Drawing for the job (mm, zero at the part's lowest x, y, z). A direction names the side the tool comes from. Give positions to 0.01 mm unless a question says otherwise; leave off trailing zeros. Order: outer loops, then holes, each group sorted by start corner. A loop starts at its lowest first (then second) coordinate and runs counter-clockwise, first axis right, second up. Notation, with made-up numbers: (-24.5, -40) -> (-3.5, -40) arc R25 cw to (-3.5, -20) -> close; hole circle Ø5 at (4, 65). An arc over 180 degrees is marked (long way). One line per item, written item: value. Start each with the question number.
(1) Pin check, flat tips, straight feed: pin 1 (17.5 mm diameter, centred on x = 24, z = 24.5, fed in from +Y); pin 2 (6.5 mm diameter, centred on x = 40.5, y = 7.5, fed in from +Z); pin 3 (4.5 mm diameter, centred on x = 7.5, y = 7.5, fed in from -Z); pin 4 (7.5 mm diameter, centred on y = 5, z = 12, fed in from -X). Stop position of each tip, or through.
(2) Saw through at D-D on x = 7.5. Give the cut face in (y, z), plus the area to 3 significant figures.
(3) Probe line 1 (Y direction, x = 40.5, z = 3.35); line 2 (Z direction, x = 24, y = 9); line 3 (Y direction, x = 40, z = 3). List the from-to ranges inside material, lowest first.
(4) Saw through at A-A on y = 43.5. Give the cut face in (x, z), plus the area to 3 significant figures.
(5) Which spindle directions (+Z, -Z, +X, -X, +Y, -Y) get a long thin tool onto all of the face, cutting with end or side? Do the marked faces 1, 2, 3, 4 and 5. Say none if no direction does.
(6) Two-plate mould, pull along X, no slides. Class the marked faces 6, 7 and 8: +X half, -X half, draft (parallel to the pull), parting line (faces both ways), or undercut.
(7) Saw through at C-C on x = 24. Give the cut face in (y, z), plus the area to 4 significant figures.
(8) Saw through at B-B on z = 28. Give the cut face in (x, y), plus the area to 3 significant figures.
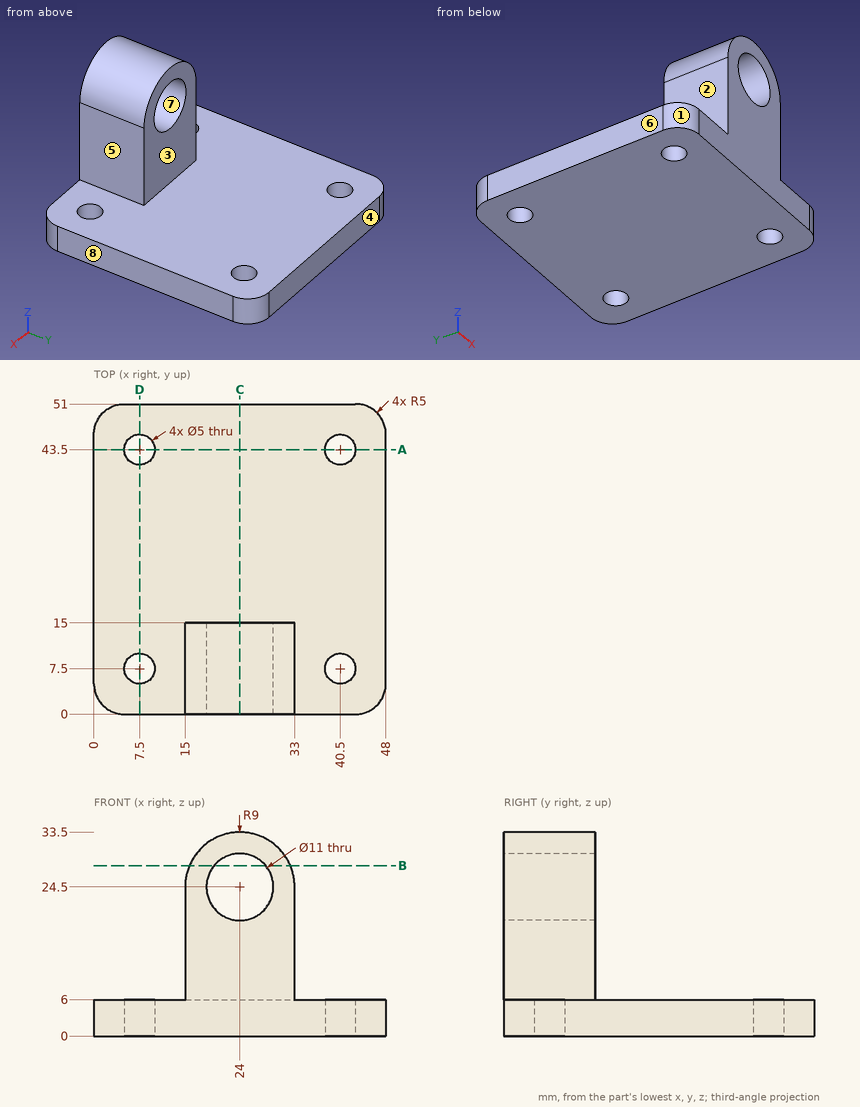
Results below:
1. pin 1: stops at y = 15
1. pin 2: stops at z = 6
1. pin 3: passes through
1. pin 4: stops at x = 15
2. outline: (0, 0) -> (5, 0) -> (5, 6) -> (0, 6) -> close; (10, 0) -> (41, 0) -> (41, 6) -> (10, 6) -> close; (46, 0) -> (51, 0) -> (51, 6) -> (46, 6) -> close
2. area: 246 mm²
3. line 1: y = 0 to 5, 10 to 41, 46 to 51
3. line 2: z = 0 to 19, 30 to 33.5
3. line 3: y = 0 to 5.05, 9.95 to 41.05, 45.95 to 51
4. outline: (0, 0) -> (5, 0) -> (5, 6) -> (0, 6) -> close; (10, 0) -> (38, 0) -> (38, 6) -> (10, 6) -> close; (43, 0) -> (48, 0) -> (48, 6) -> (43, 6) -> close
4. area: 228 mm²
5. face 1: +Z, -Z, -X, -Y
5. face 2: +Z, -X, +Y, -Y
5. face 3: +Z, +X, -X, +Y
5. face 4: +Z, -Z, +X, -X, +Y
5. face 5: +Z, +X, +Y, -Y
6. face 6: -X half
6. face 7: undercut
6. face 8: +X half
7. outline: (0, 0) -> (51, 0) -> (51, 6) -> (15, 6) -> (15, 19) -> (0, 19) -> close; (0, 30) -> (15, 30) -> (15, 33.5) -> (0, 33.5) -> close
7. area: 553.5 mm²
8. outline: (15.71, 0) -> (19.76, 0) -> (19.76, 15) -> (15.71, 15) -> close; (28.24, 0) -> (32.29, 0) -> (32.29, 15) -> (28.24, 15) -> close
8. area: 121 mm²
